Model file for the job. Use its own axes, mm. A direction names the side the tool comes from. Give positions to 0.01 mm unless a question says otherwise; leave off trailing zeros. Loops run counter-clockwise (first coordinate to the right, second up) from the corner with the lowest first, then second, coordinate; pieces in that order, holes last. Notation, with made-up numbers: M 6,62 L 13,62 A18 cw 13,89 Z; hole C 14,33.25 d3. An arc over 180 degrees is marked long. Answer in a Markdown table with one row per item.
```python
from build123d import *

# Parameters (mm, degrees)
SKETCH_1_R          = 5
SKETCH_1_R_2        = 2.5
EXTRUDE_1_DEPTH     = 3
SKETCH_3_R          = 2.5
EXTRUDE_2_DEPTH     = 15
SKETCH_4_W          = 25
SKETCH_4_H          = 12
CUT_EXTRUDE_1_DEPTH = 10
FILLET_1_R          = 2


with BuildPart() as part:
    # 스케치1 → 보스-돌출1 (new body)
    with BuildSketch(Plane.XY):
        with BuildLine():
            ThreePointArc((-31.622776602, -15), (35, 0), (-31.622776602, 15))
            Line((-31.622776602, 15), (-63.245553203, 15))
            ThreePointArc((-63.245553203, 15), (-65, 0), (-63.245553203, -15))
            Line((-63.245553203, -15), (-31.622776602, -15))
        make_face()
        with BuildLine():
            ThreePointArc((-13.750000001, -23.815698604), (-12.834936371, -27.230761907), (-16.249999587, -28.145825861))
            ThreePointArc((-16.249999587, -28.145825861), (-32.5, -2.35e-07), (-16.249999995, 28.145825626))
            ThreePointArc((-16.249999995, 28.145825626), (-12.834936369, 27.230761903), (-13.750000416, 23.815698364))
            ThreePointArc((-13.750000416, 23.815698364), (-27.5, -2.4e-07), (-13.750000001, -23.815698604))
        make_face(mode=Mode.SUBTRACT)
        Circle(SKETCH_1_R, mode=Mode.SUBTRACT)
        with Locations((-55, 0)):
            Circle(SKETCH_1_R_2, mode=Mode.SUBTRACT)
    extrude(amount=EXTRUDE_1_DEPTH)

    # 스케치3 → 보스-돌출2 (add, symmetric)
    with BuildSketch(Plane(origin=(0, 0, 0), x_dir=(1, 0, 0), z_dir=(0, 1, 0))):
        with BuildLine():
            Line((-10, 0), (10, 0))
            Line((10, 0), (5.262640911, 15.598314937))
            ThreePointArc((5.262640911, 15.598314937), (0, 19.5), (-5.262640911, 15.598314937))
            Line((-5.262640911, 15.598314937), (-10, 0))
        make_face()
        with Locations(Location((0, 14, 0), (0, 0, 270))):
            Circle(SKETCH_3_R, mode=Mode.SUBTRACT)
    extrude(amount=EXTRUDE_2_DEPTH, both=True)

    # 스케치4 → 컷-돌출1 (cut, symmetric)
    with BuildSketch(Plane(origin=(0, 0, 0), x_dir=(0, 0, -1), z_dir=(1, 0, 0))):
        with Locations((12.5, 0)):
            Rectangle(SKETCH_4_W, SKETCH_4_H)
    extrude(amount=CUT_EXTRUDE_1_DEPTH, both=True, mode=Mode.SUBTRACT)

    # 필렛1
    fillet_1_edges = [part.edges().sort_by_distance(p)[0] for p in [
        (-5, 0, 3),
    ]]
    fillet(fillet_1_edges, radius=FILLET_1_R)


solid = part.part
```
Q1. Saw through at D-D (z = -2.25). Give the cut face in (x, y).
Reported:
| item | result |
|---|---|
| outline | M -9.32,-15 L 9.32,-15 L 9.32,-6 L -9.32,-6 Z; M -9.32,6 L 9.32,6 L 9.32,15 L -9.32,15 Z |
Q2. 3-axis set-ups, long thin cutter, end or side, ignore diameter. For faces 5 (the face through (-48, -15, 1)), 6 (the face through (0, 15, -8)), 7 (the face through (7.664, -10.437, -7.69)), 8 (the face through (0, -15, -8)), 9 (the face through (-32.497, -0.476, 1.479)): which of +Z, -Z, +X, -X, +Y, -Y reach the whole face in a straight line?
Reported:
| item | result |
|---|---|
| face 5 | +Z, -Z, -X, -Y |
| face 6 | -Z, +X, -X, +Y |
| face 7 | -Z, +X, +Y, -Y |
| face 8 | -Z, +X, -X, -Y |
| face 9 | +Z, -Z |
Q3. Saw through at C-C (x = -55). Give the cut face in (y, z), and give its area (3 significant figures).
Reported:
| item | result |
|---|---|
| outline | M -15,0 L -2.5,0 L -2.5,3 L -15,3 Z; M 2.5,0 L 15,0 L 15,3 L 2.5,3 Z |
| area | 75.0 mm² |
Q4. Drop flat-ended pins along their axis: pin 1 (5 mm diameter, centred on y = -9.5, z = -7.5, fed in from +X); pin 2 (10 mm diameter, centred on x = -0.5, z = -8, fed in from +Y); pin 3 (10 mm diameter, centred on x = -2, z = -14, fed in from -Y). Give the stop position or say it passes through.
Reported:
| item | result |
|---|---|
| pin 1 | x = 8.48 |
| pin 2 | y = 15 |
| pin 3 | y = -15 |
Q5. Saw through at A-A (x = 0). Give the cut face in (y, z), and give its area (3 significant figures).
Reported:
| item | result |
|---|---|
| outline | M -35,0 L -15,0 L -15,-11.5 L -6,-11.5 L -6,0 L -5,0 L -5,1 A2 ccw -7,3 L -35,3 Z; M -15,-19.5 L -6,-19.5 L -6,-16.5 L -15,-16.5 Z; M 5,0 L 6,0 L 6,-11.5 L 15,-11.5 L 15,0 L 35,0 L 35,3 L 7,3 A2 ccw 5,1 Z; M 6,-19.5 L 15,-19.5 L 15,-16.5 L 6,-16.5 Z |
| area | 439 mm² |
Q6. Mould opens along Y. For faces 1 (the face through (0, -6, -7)), 2 (the face through (-47, 15, 1)), 3 (the face through (-7.6, -10.4, -7.9)), 4 (the face through (-12.808, -27.183, 1.479)) say: released by +Y, released by -Y, zero draft, split by the parting line, or undercut.
Reported:
| item | result |
|---|---|
| face 1 | undercut |
| face 2 | released by +Y |
| face 3 | zero draft |
| face 4 | undercut |
Q7. Probe probe 1 along Y at (x, z) = (0, 0.6); probe 2 along Z at (x, y) = (6, -30.5); probe 3 along Y at (x, z) = (-55, 1.25). List the from-to ranges inside material, lowest first.
Reported:
| item | result |
|---|---|
| probe 1 | -35 to -5, 5 to 35 |
| probe 2 | 0 to 3 |
| probe 3 | -15 to -2.5, 2.5 to 15 |
Q8. Saw through at B-B (y = 0). Give the cut face in (x, z), and give its area (3 significant figures).
Reported:
| item | result |
|---|---|
| outline | M -65,0 L -57.5,0 L -57.5,3 L -65,3 Z; M -52.5,0 L -32.5,0 L -32.5,3 L -52.5,3 Z; M -27.5,0 L -5,0 L -5,1 A2 ccw -7,3 L -27.5,3 Z; M 5,0 L 35,0 L 35,3 L 7,3 A2 ccw 5,1 Z |
| area | 238 mm² |
